Source: CAD feature listing. Evaluate the final solid. Frame: model axes, mm. Face numbers are marked on the shaded views. A direction names the side the tool comes from. Give positions to 0.01 mm unless a question says otherwise; leave off trailing zeros. Loops run counter-clockwise (first coordinate to the right, second up) from the corner with the lowest first, then second, coordinate; pieces in that order, holes last. Notation, with made-up numbers: M 58,12.25 L 70,12.25 A11 cw 70,27.25 Z; hole C 82,53 d6. An arc over 180 degrees is marked long. Answer in a Markdown table with one row per item.
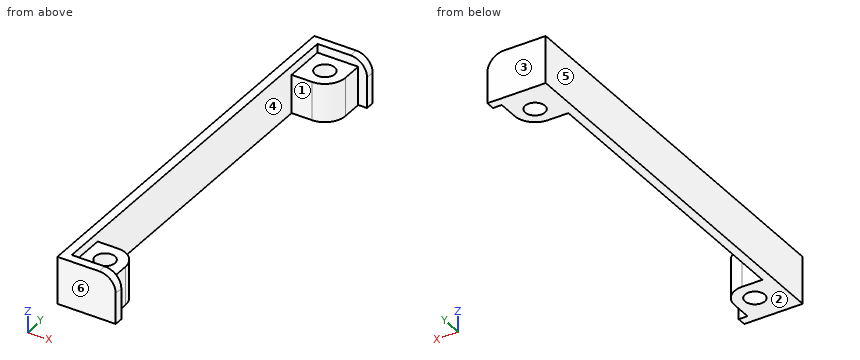
```python
from build123d import *

# Parameters (mm, degrees)
SKETCH_1_R        = 1.8
EXTRUDE_1_DEPTH   = 7
EXTRUDE_1_2_DEPTH = 7
EXTRUDE_2_DEPTH   = 8.6
FILLET_1_R        = 3


with BuildPart() as part:
    # Sketch 1 → Extrude 1 (new body)
    with BuildSketch(Plane.XY):
        with BuildLine():
            Line((1.6, 1.6), (9, 1.6))
            Line((9, 1.6), (9, 5.3))
            ThreePointArc((9, 5.3), (7.91629509, 7.91629509), (5.3, 9))
            Line((5.3, 9), (1.6, 9))
            Line((1.6, 9), (1.6, 1.6))
        make_face()
        with Locations((5.3, 5.3)):
            Circle(SKETCH_1_R, mode=Mode.SUBTRACT)
    extrude(amount=EXTRUDE_1_DEPTH)



with BuildPart() as body_2:
    # Sketch 1 → Extrude 1 2 (new body)
    with BuildSketch(Plane.XY):
        with BuildLine():
            Line((1.6, 71.865), (1.6, 64.465))
            Line((1.6, 64.465), (5.3, 64.465))
            ThreePointArc((5.3, 64.465), (7.91629509, 65.54870491), (9, 68.165))
            Line((9, 68.165), (9, 71.865))
            Line((9, 71.865), (1.6, 71.865))
        make_face()
        with Locations((5.3, 68.165)):
            Circle(SKETCH_1_R, mode=Mode.SUBTRACT)
    extrude(amount=EXTRUDE_1_2_DEPTH)


with BuildPart() as part_1:
    add(part.part)

    add(body_2.part)  # Extrude 2 merges body 2
    # Sketch 1_3 → Extrude 2 (add)
    with BuildSketch(Plane.XY):
        Polygon((0, 73.465), (0, 0), (10.6, 0), (10.6, 1.6), (1.6, 1.6), (1.6, 71.865), (10.6, 71.865), (10.6, 73.465), align=None)
    extrude(amount=EXTRUDE_2_DEPTH)

    # Fillet 1
    fillet_1_edges = [part_1.edges().sort_by_distance(p)[0] for p in [
        (10.6, 72.665, 8.6),
        (10.6, 0.8, 8.6),
    ]]
    fillet(fillet_1_edges, radius=FILLET_1_R)


solid = part_1.part
```
Q1. Mould query, pull axis Y, two halves, no side actions, for the marked faces 3, 4, 5 and 6. Classes: +Y half, -Y half, draft (parallel to the pull), parting line (faces both ways), or undercut.
Values follow:
| item | result |
|---|---|
| face 3 | +Y half |
| face 4 | undercut |
| face 5 | draft |
| face 6 | -Y half |
Q2. Section query B-B (z = 1). Output: boundary loops of the cut face in (x, y) (3 decimals), plus the area to 3 significant figures.
Values follow:
| item | result |
|---|---|
| outline | M 0,0 L 10.6,0 L 10.6,1.6 L 9,1.6 L 9,5.3 A3.7 ccw 5.3,9 L 1.6,9 L 1.6,64.465 L 5.3,64.465 A3.7 ccw 9,68.165 L 9,71.865 L 10.6,71.865 L 10.6,73.465 L 0,73.465 Z; hole C 5.3,5.3 d3.6; hole C 5.3,68.165 d3.6 |
| area | 230 mm^2 |
Q3. Ray query, probe 1 along Y at (x, z) = (5.3, 1.75) (3 decimals); probe 2 along Y at (x, z) = (1.75, 2.5) (3 decimals); probe 3 along Y at (x, z) = (6.25, 6) (3 decimals). Return the intervals inside material, ascending. Write a range as from..to.
Values follow:
| item | result |
|---|---|
| probe 1 | 0..3.5, 7.1..9, 64.465..66.365, 69.965..73.465 |
| probe 2 | 0..9, 64.465..73.465 |
| probe 3 | 0..3.771, 6.829..8.876, 64.589..66.636, 69.694..73.465 |
Q4. Reachability of the marked faces 1 and 2 from +Z, -Z, +X, -X, +Y, -Y: full face, straight path, thin tool, end or side. Return the list, or none.
Values follow:
| item | result |
|---|---|
| face 1 | +Z, -Z, +X |
| face 2 | -Z, +X, -X, +Y, -Y |
Q5. Contact query for flat-ended pins moving along their axis: pin 1 Ø6 at (x, y) = (6, 50) entering from +Z; pin 2 Ø4.5 at (x, z) = (5, 5) entering from -Y; pin 3 Ø1.8 at (y, z) = (3, 4) entering from +X; pin 4 Ø6 at (x, y) = (5.3, 68.165) entering from +Z. Output: stop coordinate, or through.
Values follow:
| item | result |
|---|---|
| pin 1 | through |
| pin 2 | y = 0 |
| pin 3 | x = 9 |
| pin 4 | z = 7 |
Q6. Section query D-D (y = 35). Output: boundary loops of the cut face in (x, z).
Values follow:
| item | result |
|---|---|
| outline | M 0,0 L 1.6,0 L 1.6,8.6 L 0,8.6 Z |
Q7. Section query A-A (x = 10). Output: boundary loops of the cut face in (y, z) (3 decimals), plus the area to 3 significant figures.
Values follow:
| item | result |
|---|---|
| outline | M 0,0 L 1.6,0 L 1.6,7.4 L 0,7.4 Z; M 71.865,0 L 73.465,0 L 73.465,7.4 L 71.865,7.4 Z |
| area | 23.7 mm^2 |
Q8. Section query C-C (x = 4.25). Output: boundary loops of the cut face in (y, z) (3 decimals).
Values follow:
| item | result |
|---|---|
| outline | M 0,0 L 3.838,0 L 3.838,7 L 1.6,7 L 1.6,8.6 L 0,8.6 Z; M 6.762,0 L 9,0 L 9,7 L 6.762,7 Z; M 64.465,0 L 66.703,0 L 66.703,7 L 64.465,7 Z; M 69.627,0 L 73.465,0 L 73.465,8.6 L 71.865,8.6 L 71.865,7 L 69.627,7 Z |
